Work out the finished part from the listing and answer in its coordinate system (mm). A direction names the side the tool comes from. Coordinates: 2 decimals unless noted, no trailing zeros. Write each loop counter-clockwise with the first axis right and the second up, starting at its lowest first coordinate (ties: lowest second). Pieces come first, ordered by that corner, then holes. Notation, with made-up numbers: (-21, 87) - (-15, 87) arc R37 ccw to (-15, 123) - close; hole circle Ø11 at (12.5, 73). An arc over 180 degrees is marked (long way). Use one line per item in the form item = value. Start each with the question number.
Item 1: A cutting plane is placed at A-A (y = 0). Write down the section's boundary in (x, z).
Item 2: Determine the mould class of faces 3 (the flat face through (-1.5, -53, 1)), 4 (the cylindrical face through (-67.883, 31.888, 1.479)), 5 (the flat face through (-17, -37, 3)), 6 (the flat face through (61.84, 27.18, 1.48)) for opening direction Y: released by +Y, released by -Y, zero draft, split by the parting line, or undercut.
Item 3: Given pin 1 (1.5 mm diameter, centred on y = -53.5, z = 1.5, fed in from -X); pin 2 (0.9 mm diameter, centred on x = -0.5, z = 1, fed in from -Y); pin 3 (1.5 mm diameter, centred on x = -38.5, z = 0.5, fed in from -Y), each flat-ended and moving along its own axis, determine where each tip first touches the part or whether it passes through.
Item 4: A cutting plane is placed at C-C (z = 0.45). Give the number of separate pieces and of enclosed holes in the cut face, then the cut area to 3 significant figures.
Item 5: For faces 1 (the cylindrical face through (0, -75, 1)), 2 (the flat face through (46.98, 23.56, 1.48)), determine the directions among +Z, -Z, +X, -X, +Y, -Y from which every point of the face is accessible in a straight line to the end or side of a thin tool.
Item 6: A cutting plane is placed at B-B (x = 33). Write down the section's boundary in (y, z).
Item 7: Consider probe 1 along X at (y, z) = (23, 2.5); probe 2 along Y at (x, z) = (-32.5, 2.6); probe 3 along X at (y, z) = (15, 2.5). Determine where each line is inside the solid, lowest interval first.
from build123d import *

# Parameters (mm, degrees)
SKETCH1_R           = 40
SKETCH1_R_2         = 1.15
SKETCH1_R_3         = 1.5
SKETCH1_W           = 3
SKETCH1_H           = 5
BOSS_EXTRUDE1_DEPTH = 3


with BuildPart() as part:
    # Sketch1 → Boss-Extrude1 (new body)
    with BuildSketch(Plane.XY):
        with BuildLine():
            Line((-72.939022771, 17.461356112), (-10, -74.330343737))
            ThreePointArc((-10, -74.330343737), (0, -75), (10, -74.330343737))
            Line((10, -74.330343737), (72.939022771, 17.461356112))
            ThreePointArc((72.939022771, 17.461356112), (67.973084028, 31.696369631), (60.260474918, 44.650589723))
            Line((60.260474918, 44.650589723), (-60.260474918, 44.650589723))
            ThreePointArc((-60.260474918, 44.650589723), (-67.973084028, 31.696369631), (-72.939022771, 17.461356112))
        make_face()
        Circle(SKETCH1_R, mode=Mode.SUBTRACT)
        with Locations((0, -43)):
            Circle(SKETCH1_R_2, mode=Mode.SUBTRACT)
        with Locations((-37.239092363, -21.5)):
            Circle(SKETCH1_R_2, mode=Mode.SUBTRACT)
        with Locations((-37.239092363, 21.5)):
            Circle(SKETCH1_R_2, mode=Mode.SUBTRACT)
        with Locations((0, 43)):
            Circle(SKETCH1_R_2, mode=Mode.SUBTRACT)
        with Locations((37.239092363, 21.5)):
            Circle(SKETCH1_R_2, mode=Mode.SUBTRACT)
        with Locations((37.239092363, -21.5)):
            Circle(SKETCH1_R_2, mode=Mode.SUBTRACT)
        with Locations((0, -60)):
            Circle(SKETCH1_R_3, mode=Mode.SUBTRACT)
        with Locations((54.378467222, 25.357095704)):
            Circle(SKETCH1_R_3, mode=Mode.SUBTRACT)
        with Locations((-54.378467222, 25.357095704)):
            Circle(SKETCH1_R_3, mode=Mode.SUBTRACT)
        with Locations((0, -52.5)):
            Rectangle(SKETCH1_W, SKETCH1_H, mode=Mode.SUBTRACT)
        with Locations((0, -67.5)):
            Rectangle(SKETCH1_W, SKETCH1_H, mode=Mode.SUBTRACT)
        Polygon((49.213000894, 24.603466076), (44.681461959, 22.490374768), (45.949316744, 19.771451406), (50.48085568, 21.884542715), align=None, mode=Mode.SUBTRACT)
        Polygon((58.276078765, 28.829648694), (62.8076177, 30.942740002), (64.075472485, 28.223816641), (59.54393355, 26.110725333), align=None, mode=Mode.SUBTRACT)
        Polygon((-58.276078765, 28.829648694), (-62.8076177, 30.942740002), (-64.075472485, 28.223816641), (-59.54393355, 26.110725333), align=None, mode=Mode.SUBTRACT)
        Polygon((-49.213000894, 24.603466076), (-44.681461959, 22.490374768), (-45.949316744, 19.771451406), (-50.48085568, 21.884542715), align=None, mode=Mode.SUBTRACT)
    extrude(amount=BOSS_EXTRUDE1_DEPTH)


solid = part.part
Answer:
q1.outline = (-60.97, 0) - (-40, 0) - (-40, 3) - (-60.97, 3) - close; (40, 0) - (60.97, 0) - (60.97, 3) - (40, 3) - close
q2.face_3 = undercut
q2.face_4 = released by +Y
q2.face_5 = zero draft
q2.face_6 = undercut
q3.pin_1 = -24.8
q3.pin_2 = -75
q3.pin_3 = -33.86
q4.separate_pieces = 1
q4.enclosed_holes = 16
q4.area = 6,140 mm²
q5.face_1 = +Z, -Z, -Y
q5.face_2 = +Z, -Z
q6.outline = (-40.79, 0) - (-22.61, 0) - (-22.61, 3) - (-40.79, 3) - close; (22.61, 0) - (44.65, 0) - (44.65, 3) - (22.61, 3) - close
q7.probe_1 = -71.39 to -49.96, -45.77 to -32.73, 32.73 to 45.77, 49.96 to 71.39
q7.probe_2 = -41.52 to -23.32, 23.32 to 44.65
q7.probe_3 = -71.25 to -37.08, 37.08 to 71.25
